The model under review builds one solid part; all positions refer to its coordinate system, in mm. A direction names the side the tool comes from. Coordinates: 2 decimals unless noted, no trailing zeros. Write each loop counter-clockwise with the first axis right and the second up, starting at its lowest first coordinate (ties: lowest second). Pieces come first, ordered by that corner, then holes. Notation, with made-up numbers: (37, 83.25) -> (60, 83.25) arc R28 cw to (60, 113.25) -> close; hole circle Ø10 at (86.25, -13). An arc over 180 degrees is marked (long way). Write each question's results on one line, items separated by ' | '.
Solid Edge part; units mm, degrees
sketch "Sketch1" plane through (0, 0, 0) normal (0, -1, 0) x (1, 0, 0)
  line L0 (2.5, 0) -> (5, 2.5)
  line L1 (5, 2.5) -> (5, 2.8)
  line L2 (5, 2.8) -> (0, 2.8)
  line L3 (0, 2.8) -> (0, -13.2)
  line L4 (0, -13.2) -> (2.0095, -13.2)
  line L5 (2.0095, -13.2) -> (2.5, -12.7095)
  line L6 (2.5, -12.7095) -> (2.5, -2.4)
  line L7 (2.5, -2.4) -> (2.0095, -2.4)
  line L8 (2.0095, -2.4) -> (2.0095, -2.39)
  line L9 (2.0095, -2.39) -> (2.5, -2.39)
  line L10 (2.5, -2.39) -> (2.5, 0)
  dimension "D1" = 2.5
  dimension "D2" = 2.0095
revolve "RevolvedProtrusion1" add sketch "Sketch1" angle 360 about axis through (0, 0, 54) along (0, 0, -1)
sketch "Sketch2" plane through (0, 0, 0) normal (0, -1, 0) x (1, 0, 0)
  arc A0 (-1.5, 0.5) -> (0, 0) centre (0, 2.5) ccw
  line L0 (0, 0.5) -> (0, 0)
  line L1 (-1.5, 0.5) -> (0, 0.5)
revolve "RevolvedCutout1" cut sketch "Sketch2" angle 360 about axis through (0, 0, 54) along (0, 0, -1)
sketch "Sketch3" plane through (0, 0, 2.8) normal (0, 0, 1) x (0, -1, 0)
  line L0 (-1.7321, 0) -> (-0.866, 1.5)
  line L1 (-0.866, 1.5) -> (0.866, 1.5)
  line L2 (0.866, 1.5) -> (1.7321, 0)
  line L3 (1.7321, 0) -> (0.866, -1.5)
  line L4 (0.866, -1.5) -> (-0.866, -1.5)
  line L5 (-0.866, -1.5) -> (-1.7321, 0)
extrude "Cutout1" cut sketch "Sketch3" against normal blind 2.3
cosmetic_thread "Thread1"
sketch "Sketch4" plane through (0, 0, 0) normal (1, 0, 0) x (0, 1, 0)
  line L0 (-1.72, 2.8) -> (0, 1.807)
revolve "RevolvedCutout2" cut sketch "Sketch4" angle 360 about axis through (0, 0, -57) along (0, 0, 1) material side at (0, -0.835, 2.3468)
fillet "Round1" radius 0.2 1 edges at (-2.5, 0, 0)
properties material "Stahl"
Q1. Add section A-A (z = 1.5). Write out the cut boundary in (x, y), plus the area to 3 significant figures.
Solution:
outline: circle Ø8 at (0, 0); hole (-1.5, -0.87) -> (0, -1.73) -> (1.5, -0.87) -> (1.5, 0.87) -> (0, 1.73) -> (-1.5, 0.87) -> close | area: 42.5 mm²
Q2. For line 1 (X direction, y = -2, z = -7.75); line 2 (Z direction, x = 0, y = -3), list the stretches that pass through material, from the lowest coordinate up. Write a range as from..to.
Solution:
line 1: -1.5..1.5 | line 2: 0.5..2.8
Q3. Add section B-B (z = -1). Write out the cut boundary in (x, y).
Solution:
outline: circle Ø5 at (0, 0)
Q4. Machinability: for faces 4 (the cylindrical face through (4.77, 1.5, 2.65)), 5 (the flat face through (0.76, -1.293, 1.666)), which of the approach directions +Z, -Z, +X, -X, +Y, -Y give a long, thin tool a straight path to every point of the face, cutting with its end or side? Answer none if there is none.
Solution:
face 4: +Z, -Z | face 5: +Z
Q5. Draft analysis for pull direction Z (two halves, no side actions). For faces 1 (the flat face through (0, 0, -13.2)), 2 (the flat face through (2, 0, 2.8)), 3 (the flat face through (-0.76, 1.293, 1.666)), state which applies: pulls with the +Z half, pulls with the -Z half, needs draft (parallel to the pull), parting line crosses it, or undercut.
Solution:
face 1: pulls with the -Z half | face 2: pulls with the +Z half | face 3: needs draft
Q6. Clearance check with flat-ended pins moving along their axes: P1, Ø4, axis at y = -2.5, z = -4.5, coming from the +X side; P2, Ø1.9, axis at y = -0.5, z = 1, coming from the -X side; P3, Ø3, axis at y = 3, z = -8.5, coming from the -X side. State where each tip first meets the part, or that it passes through.
Solution:
P1: x = 2.45 | P2: x = -4.43 | P3: x = -2
